```python
from build123d import *

# Parameters (mm, degrees)
F0_W     = 20
F0_H     = 30
F1_DEPTH = 2
F2_R     = 2
F3_W     = 17
F3_H     = 27
F4_DEPTH = 5
F5_R     = 2
F6_SIZE  = 0.5
F7_R     = 0.5


with BuildPart() as f1:
    # F0 (on Top) → F1 (new body)
    with BuildSketch(Plane.XY):
        Rectangle(F0_W, F0_H)
    extrude(amount=F1_DEPTH)

    # F2
    f2_edges = [f1.edges().sort_by_distance(p)[0] for p in [
        (-10, -15, 1),
        (10, -15, 1),
        (-10, 15, 1),
        (10, 15, 1),
    ]]
    fillet(f2_edges, radius=F2_R)

    # F3 (on face) → F4 (join)
    with BuildSketch(Plane.XY.offset(2)):
        Rectangle(F3_W, F3_H)
    extrude(amount=F4_DEPTH)

    # F5
    f5_edges = [f1.edges().sort_by_distance(p)[0] for p in [
        (-8.5, -13.5, 4.5),
        (8.5, -13.5, 4.5),
        (-8.5, 13.5, 4.5),
        (8.5, 13.5, 4.5),
    ]]
    fillet(f5_edges, radius=F5_R)

    # F6
    f6_edges = [f1.edges().sort_by_distance(p)[0] for p in [
        (-8.5, 0, 7),
    ]]
    chamfer(f6_edges, length=F6_SIZE)

    # F7
    f7_edges = [f1.edges().sort_by_distance(p)[0] for p in [
        (0, 15, 0),
        (9.414214, 14.414214, 0),
        (-9.414214, 14.414214, 0),
        (10, 0, 0),
        (-10, 0, 0),
        (9.414214, -14.414214, 0),
        (-9.414214, -14.414214, 0),
        (0, -15, 0),
    ]]
    fillet(f7_edges, radius=F7_R)


solid = f1.part
```
Part model, mm, in its own coordinate system. A direction names the side the tool comes from. Coordinates: 2 decimals unless noted, no trailing zeros. Order: outer loops, then holes, each group sorted by start corner. A loop starts at its lowest first (then second) coordinate and runs counter-clockwise, first axis right, second up. Notation, with made-up numbers: (-12, 43.5) - (11, 43.5) arc R19 ccw to (11, 51.5) - close; hole circle Ø7 at (53, 41.25). An arc over 180 degrees is marked (long way). Return JSON: item names as keys, results as strings. Group by question number.
Item 1: Cut at B-B (x = -6). List the corners of the cut face in (y, z).
Item 2: Which spindle directions (+Z, -Z, +X, -X, +Y, -Y) get a long thin tool onto all of the face, cutting with end or side? Do faces 1 (the face through (-7.9, -12.93, 4.28)), 2 (the face through (0, -13.5, 4)), 3 (the face through (-7.9, 12.93, 4.28)). Say none if no direction does.
Item 3: Drill centre lines: probe 1 along X at (y, z) = (-11, 5.5); probe 2 along Y at (x, z) = (1, 5.75); probe 3 along Z at (x, y) = (-8.75, 14). Where is each one in solid material? Low to high. Write a range as from..to.
Item 4: Cut at C-C (y = 10.5). List the corners of the cut face in (x, z), plus the area to 3 significant figures.
Item 5: Cut at A-A (z = 5). List the corners of the cut face in (x, y).
Item 6: Pin check, flat tips, straight feed: pin 1 (1.3 mm diameter, centred on x = 2, z = 4, fed in from -Y); pin 2 (3.5 mm diameter, centred on y = -4, z = 4.5, fed in from -X). Stop position of each tip, or through.
Check values:
{
 "1": {"outline": "(-15, 0.5) arc R0.5 ccw to (-14.5, 0) - (14.5, 0) arc R0.5 ccw to (15, 0.5) - (15, 2) - (13.5, 2) - (13.5, 6.5) - (13, 7) - (-13, 7) - (-13.5, 6.5) - (-13.5, 2) - (-15, 2) - close"},
 "2": {"face 1": "+Z, -X, -Y", "face 2": "+Z, +X, -X, -Y", "face 3": "+Z, -X, +Y"},
 "3": {"probe 1": "x = -8.5..8.5", "probe 2": "y = -13.5..13.5", "probe 3": "z = 0..2"},
 "4": {"outline": "(-10, 0.5) arc R0.5 ccw to (-9.5, 0) - (9.5, 0) arc R0.5 ccw to (10, 0.5) - (10, 2) - (8.5, 2) - (8.5, 6.5) - (8, 7) - (-8, 7) - (-8.5, 6.5) - (-8.5, 2) - (-10, 2) - close", "area": "125 mm2"},
 "5": {"outline": "(-8.5, -11.5) arc R2 ccw to (-6.5, -13.5) - (6.5, -13.5) arc R2 ccw to (8.5, -11.5) - (8.5, 11.5) arc R2 ccw to (6.5, 13.5) - (-6.5, 13.5) arc R2 ccw to (-8.5, 11.5) - close"},
 "6": {"pin 1": "stops at y = -13.5", "pin 2": "stops at x = -8.5"}
}
